Can you work these out from the model? Positions are in its coordinate system, mm. A direction names the side the tool comes from. Round coordinates to 2 decimals unless told otherwise and drop trailing zeros. Loops run counter-clockwise (first coordinate to the right, second up) from the corner with the lowest first, then second, coordinate; pieces in that order, holes last.
```python
from build123d import *

# Parameters (mm, degrees)
F1_DEPTH = 63.5
F0_W     = 25.4
F0_H     = 19.05
F2_DEPTH = 25.4
F3_DEPTH = 10.4775
F5_R     = 6.35
F7_D     = 25.4


with BuildPart() as f1:
    # F0 (on Front) → F1 (new body, symmetric)
    with BuildSketch(Plane.XZ):
        Polygon((-41.275, 9.525), (-41.275, -9.525), (41.275, -9.525), (41.275, 9.525), (22.225, 9.525), align=None)
    extrude(amount=F1_DEPTH, both=True)

    # F0 (on Front) → F2 (join, symmetric)
    with BuildSketch(Plane.XZ):
        with Locations((73.025, 52.4002)):
            Rectangle(F0_W, F0_H)
        with BuildLine():
            Line((22.225, 9.525), (41.275, 9.525))
            Line((41.275, 9.525), (41.275, 27.0002))
            ThreePointArc((41.275, 27.0002), (45.9246798487, 38.2255201513), (57.15, 42.8752))
            Line((57.15, 42.8752), (60.325, 42.8752))
            Line((60.325, 42.8752), (60.325, 61.9252))
            Line((60.325, 61.9252), (57.15, 61.9252))
            add(Edge.make_bspline(
                [(56.3268874615, 61.9154990929), (56.6009974392, 61.9194787375), (56.8753697614, 61.9227139639), (57.15, 61.9252)],
                knots=[110.9401343826, 110.9401343826, 110.9401343826, 110.9401343826, 111.5045361635, 111.5045361635, 111.5045361635, 111.5045361635], degree=3))
            ThreePointArc((56.3268874615, 61.9154990929), (32.1649761817, 51.4031549399), (22.225, 27.0002))
            Line((22.225, 27.0002), (22.225, 9.525))
        make_face()
    extrude(amount=F2_DEPTH, both=True)

    # F0 (on Front) → F3 (join, symmetric)
    with BuildSketch(Plane.XZ):
        with BuildLine():
            add(Edge.make_bspline(
                [(-41.275, 9.525), (-41.296369644, 31.5891025492), (2.4471890111, 61.1332508534), (56.3268874615, 61.9154990929)],
                knots=[0, 0, 0, 0, 110.9401343826, 110.9401343826, 110.9401343826, 110.9401343826], degree=3))
            Line((-41.275, 9.525), (22.225, 9.525))
            Line((22.225, 9.525), (22.225, 27.0002))
            ThreePointArc((22.225, 27.0002), (32.1649761817, 51.4031549399), (56.3268874615, 61.9154990929))
        make_face()
    extrude(amount=F3_DEPTH, both=True)

    # F0 (on Front) → F4 (revolve)
    with BuildSketch(Plane.XZ):
        Polygon((85.725, 66.675), (85.725, 61.9252), (85.725, 42.8752), (85.725, 38.1), (111.125, 38.1), (111.125, 66.675), align=None)
    revolve(axis=Axis((85.725, 0, 52.3875), (0, 0, 1)))

    # F5
    f5_edges = [f1.edges().sort_by_distance(p)[0] for p in [
        (-41.275, -63.5, 0),
        (41.275, -63.5, 0),
        (41.275, 63.5, 0),
        (-41.275, 63.5, 0),
    ]]
    fillet(f5_edges, radius=F5_R)

    # F7 (through all)
    with Locations(Plane.XY.offset(66.675)):
        with Locations((85.725, 0)):
            Hole(F7_D / 2)


solid = f1.part
```
(1) Suppose I cut it at B-B (y = 41). Write out the boundary of the cut face in (x, z) (3 decimals), then the cut area to 3 significant figures.
(2) Which directions (+Z, -Z, +X, -X, +Y, -Y) give clear straight access to the entire face, cutting with the end or side of a thin tool? Please do faces 4 (the cylindrical face through (39.464, -61.59, 0.133)), 5 (the flat face through (22.225, 18, 18)), 6 (the flat face through (41.275, -1, 4)), 7 (the flat face through (22.225, -18, 18)), 8 (the flat face through (60, 2, 42.875)).
(3) We'd pull the mould along X, two halves only. Please class faces 1 (the cylindrical face through (-39.464, 61.59, -0.133)), 2 (the flat face through (60, -2, 61.925)), 3 (the cylindrical face through (45.8, -0.4, 38.1)): released by +X, released by -X, zero draft, split by the parting line, or undercut.
(4) If I drill on line 1 (Z direction, x = 11, y = 55) (3 decimals); line 2 (Y direction, x = 15, z = 34); line 3 (X direction, y = -48, z = 0) (3 decimals), over which ranges is the centre line in solid material (lowest first)?
(5) For pin 1 (4 mm diameter, centred on y = 4, z = 19, fed in from +X) (3 decimals); pin 2 (4 mm diameter, centred on x = 13, z = 27, fed in from -Y); pin 3 (3 mm diameter, centred on y = -19, z = 39, fed in from -X), each with a flat end and sliding along its axis, tell me the tip position at first contact or that it passes through.
(6) Suppose I cut it at A-A (x = 69). Write out the boundary of the cut face in (y, z) (3 decimals).
Check result:
1. outline: (-41.275, -9.525) - (41.275, -9.525) - (41.275, 9.525) - (-41.275, 9.525) - close
1. area: 1,570 mm2
2. face 4: +Z, -Z, +X, -Y
2. face 5: +Z, -X, +Y
2. face 6: -Z, +X, +Y, -Y
2. face 7: +Z, -X, -Y
2. face 8: -Z
3. face 1: released by -X
3. face 2: zero draft
3. face 3: undercut
4. line 1: z = -9.525 to 9.525
4. line 2: y = -10.48 to 10.48
4. line 3: x = -41.275 to 41.275
5. pin 1: stops at x = 41.275
5. pin 2: stops at y = -10.48
5. pin 3: stops at x = 23.84
6. outline: (-25.4, 42.875) - (-19.116, 42.875) - (-19.116, 38.1) - (19.116, 38.1) - (19.116, 42.875) - (25.4, 42.875) - (25.4, 61.925) - (19.116, 61.925) - (19.116, 66.675) - (-19.116, 66.675) - (-19.116, 61.925) - (-25.4, 61.925) - close
